Read the model definition and answer for the solid it produces. Units are mm, in the model's axes. A direction names the side the tool comes from. Coordinates: 2 decimals unless noted, no trailing zeros. Order: outer loops, then holes, each group sorted by start corner. A loop starts at its lowest first (then second) coordinate and runs counter-clockwise, first axis right, second up. Notation, with made-up numbers: (-1, 27.5) -> (20, 27.5) arc R20 cw to (20, 54.5) -> close; hole circle Ø6 at (26, 61.5). An arc over 180 degrees is marked (long way). Use CSV: the item, a comma, the result in double quotes.
```python
from build123d import *

# Parameters (mm, degrees)
SKETCH1_R           = 17.5
SKETCH1_R_2         = 2.5
SKETCH1_R_3         = 1.75
SKETCH1_R_4         = 1
BOSS_EXTRUDE1_DEPTH = 3
FILLET1_R           = 1


with BuildPart() as part:
    # Sketch1 → Boss-Extrude1 (new body)
    # profile 1 of 13: a face of its own
    with BuildSketch(Plane.XY):
        with Locations((45.07, -38)):
            Circle(SKETCH1_R)
        with Locations((45.07, -38)):
            Circle(SKETCH1_R_2, mode=Mode.SUBTRACT)
    # profile 2 of 13: a face of its own
    with BuildSketch(Plane.XY):
        with BuildLine():
            ThreePointArc((59.178313279, -22.683979093), (56.722798651, -22.992925548), (56.413852196, -20.53741092))
            Line((56.413852196, -20.53741092), (54.366811281, -23.173695673))
            ThreePointArc((54.366811281, -23.173695673), (55.802840863, -24.177694584), (57.131272364, -25.320263845))
            Line((57.131272364, -25.320263845), (59.178313279, -22.683979093))
        make_face()
    # profile 3 of 13: a face of its own
    with BuildSketch(Plane.XY):
        with Locations((57.796082737, -21.610695007)):
            Circle(SKETCH1_R_3)
    # profile 4 of 13: a face of its own
    with BuildSketch(Plane.XY):
        with Locations((63.099282859, -27.728317587)):
            Circle(SKETCH1_R_3)
    # profile 5 of 13: a face of its own
    with BuildSketch(Plane.XY):
        with BuildLine():
            Line((62.23299639, -26.207775659), (59.33291469, -27.860016541))
            ThreePointArc((59.33291469, -27.860016541), (60.275419279, -29.337135314), (61.065487627, -30.901100396))
            Line((61.065487627, -30.901100396), (63.965569327, -29.248859515))
            ThreePointArc((63.965569327, -29.248859515), (61.578740931, -28.594604056), (62.23299639, -26.207775659))
        make_face()
    # profile 6 of 13: a face of its own
    with BuildSketch(Plane.XY):
        with BuildLine():
            ThreePointArc((65.876146235, -37.146021746), (63.921377057, -35.628168835), (65.439229968, -33.673399657))
            Line((65.439229968, -33.673399657), (62.12761863, -34.090057971))
            ThreePointArc((62.12761863, -34.090057971), (62.433110447, -35.815418664), (62.564534897, -37.56268006))
            Line((62.564534897, -37.56268006), (65.876146235, -37.146021746))
        make_face()
    # profile 7 of 13: a face of its own
    with BuildSketch(Plane.XY):
        with Locations((65.657688101, -35.409710702)):
            Circle(SKETCH1_R_3)
    # profile 8 of 13: a face of its own
    with BuildSketch(Plane.XY):
        with BuildLine():
            ThreePointArc((62.325454762, -40.915352631), (61.947425446, -42.626284719), (61.400197818, -44.29083772))
            Line((61.400197818, -44.29083772), (64.619175986, -45.173194426))
            ThreePointArc((64.619175986, -45.173194426), (63.394061913, -43.022823409), (65.54443293, -41.797709336))
            Line((65.54443293, -41.797709336), (62.325454762, -40.915352631))
        make_face()
    # profile 9 of 13: a face of its own
    with BuildSketch(Plane.XY):
        with Locations((65.081804458, -43.485451881)):
            Circle(SKETCH1_R_3)
    # profile 10 of 13: a face of its own
    with BuildSketch(Plane.XY):
        with Locations((61.459304993, -50.726082737)):
            Circle(SKETCH1_R_3)
    # profile 11 of 13: a face of its own
    with BuildSketch(Plane.XY):
        with BuildLine():
            ThreePointArc((59.896304327, -47.296811281), (58.892305416, -48.732840863), (57.749736155, -50.061272364))
            Line((57.749736155, -50.061272364), (60.386020907, -52.108313279))
            ThreePointArc((60.386020907, -52.108313279), (60.077074452, -49.652798651), (62.53258908, -49.343852196))
            Line((62.53258908, -49.343852196), (59.896304327, -47.296811281))
        make_face()
    # profile 12 of 13: a face of its own
    with BuildSketch(Plane.XY):
        with BuildLine():
            ThreePointArc((42.917509319, -55.367117892), (40.458569889, -54.881490228), (38.094226397, -54.049566432))
            Line((38.094226397, -54.049566432), (36.76608928, -58.911601248))
            ThreePointArc((36.76608928, -58.911601248), (39.141018428, -59.704773151), (41.589372203, -60.229152708))
            Line((41.589372203, -60.229152708), (42.917509319, -55.367117892))
        make_face()
    # profile 13 of 13: a face of its own
    with BuildSketch(Plane.XY):
        with BuildLine():
            ThreePointArc((41.589372203, -60.229152708), (39.141018428, -59.704773151), (36.76608928, -58.911601248))
            Line((36.76608928, -58.911601248), (32.824020556, -73.342698121))
            ThreePointArc((32.824020556, -73.342698121), (34.567840149, -76.446231348), (37.647303478, -74.660249581))
            Line((37.647303478, -74.660249581), (41.589372203, -60.229152708))
        make_face()
        with Locations((35.226677147, -74.034365596)):
            Circle(SKETCH1_R_4, mode=Mode.SUBTRACT)
    extrude(amount=BOSS_EXTRUDE1_DEPTH)

    # Fillet1
    fillet1_edges = [part.edges().sort_by_distance(p)[0] for p in [
        (62.325454762, -40.915352631, 1.5),
        (61.400197818, -44.29083772, 1.5),
        (59.896304327, -47.296811281, 1.5),
        (57.749736155, -50.061272364, 1.5),
        (54.366811281, -23.173695673, 1.5),
        (57.131272364, -25.320263845, 1.5),
        (59.33291469, -27.860016541, 1.5),
        (61.065487627, -30.901100396, 1.5),
        (62.12761863, -34.090057971, 1.5),
        (62.564534897, -37.56268006, 1.5),
    ]]
    fillet(fillet1_edges, radius=FILLET1_R)


solid = part.part
```
Item 1: Find section C-C, the plane z = 2.55. Give the number of separate pieces and of enclosed holes in the cut face, then the cut area to 3 significant figures.
Return value:
separate pieces,"1"
enclosed holes,"2"
area,"1,130 mm^2"
Item 2: Find section A-A, the plane x = 45.07. Give the vertices of the cut face in (y, z), then the cut area to 3 significant figures.
Return value:
outline,"(-55.5, 0) -> (-40.5, 0) -> (-40.5, 3) -> (-55.5, 3) -> close; (-35.5, 0) -> (-20.5, 0) -> (-20.5, 3) -> (-35.5, 3) -> close"
area,"90.0 mm^2"
Item 3: A tool of negligible diameter and unlimited length cuts with its end or side. For faces 3 (the cylindrical face through (62.525, -39.256, 1.479)), 4 (the flat face through (59.403, -51.345, 1.479)), 5 (the cylindrical face through (58.301, -26.546, 1.479)), from which of +Z, -Z, +X, -X, +Y, -Y can it reach the whole face along a straight path? Write none if from no direction.
Return value:
face 3,"+Z, -Z, +X"
face 4,"+Z, -Z, -Y"
face 5,"+Z, -Z"
Item 4: Find section D-D, the plane y = -63. Give the vertices of the cut face in (x, z), then the cut area to 3 significant figures.
Return value:
outline,"(35.65, 0) -> (40.83, 0) -> (40.83, 3) -> (35.65, 3) -> close"
area,"15.5 mm^2"
Item 5: The mould has two halves that part along Y. Classify faces 1 (the cylindrical face through (57.793, -50.393, 1.521)), 2 (the cylindrical face through (59.403, -27.534, 1.521)): +Y half, -Y half, draft (parallel to the pull), parting line (faces both ways), or undercut.
Return value:
face 1,"-Y half"
face 2,"undercut"
Item 6: Straight lines are drawn through the part: line 1 along Y through (x, z) = (45.07, 1.9); line 2 along Y through (x, z) = (64, 1.5); line 3 along Y through (x, z) = (44, 2.65). For each, find the intervals that lie inside material, in ascending order.
Return value:
line 1,"y = -55.5 to -40.5, -35.5 to -20.5"
line 2,"y = -45 to -41.37, -37.38 to -33.85, -29.23 to -26.23"
line 3,"y = -55.47 to -40.26, -35.74 to -20.53"
Item 7: Each of these flat-tipped pins is pushed along its axis until it touches: P1, Ø1.5, axis at x = 46, z = 1, coming from the +Y side; P2, Ø2.5, axis at x = 35.23, y = -74.03, coming from the +Z side; P3, Ø1, axis at y = -70.5, z = 1, coming from the +X side. Where does it stop, or does it pass through?
Return value:
P1,"stops at y = -20.5"
P2,"stops at z = 3"
P3,"stops at x = 38.92"
Item 8: Find section B-B, the plane y = -51.5. Give the vertices of the cut face in (x, z), then the cut area to 3 significant figures.
Return value:
outline,"(33.93, 0) -> (56.21, 0) -> (56.21, 3) -> (33.93, 3) -> close; (59.6, 0) -> (63.03, 0) -> (63.03, 3) -> (59.6, 3) -> close"
area,"77.1 mm^2"
